```python
from build123d import *

# Parameters (mm, degrees)
SKETCH1_R               = 16
BOSS_EXTRUDE1_DEPTH     = 25
CUT_EXTRUDE1_DEPTH      = 34.7194306
CUT_EXTRUDE1_DEPTH_BACK = 34.7194306
SKETCH2_R               = 6
CUT_EXTRUDE2_START      = -4
CUT_EXTRUDE2_DEPTH      = 12


with BuildPart() as part:
    # Sketch1 → Boss-Extrude1 (new body)
    with BuildSketch(Plane.XY):
        Circle(SKETCH1_R)
    extrude(amount=-BOSS_EXTRUDE1_DEPTH)

    # Sketch2 → Cut-Extrude1 (cut, two sides: drawn at the far end of the back side and taken through both)
    with BuildSketch(Plane(origin=(0, 0, 0), x_dir=(1, 0, 0), z_dir=(0, 1, 0)).offset(-CUT_EXTRUDE1_DEPTH_BACK)):
        with Locations(Location((0, 10, 0), (0, 0, 270))):
            Circle(SKETCH2_R)
    extrude(amount=CUT_EXTRUDE1_DEPTH + CUT_EXTRUDE1_DEPTH_BACK, mode=Mode.SUBTRACT)

    # Sketch3 → Cut-Extrude2 (cut)
    with BuildSketch(Plane.XY.offset(CUT_EXTRUDE2_START)):
        with BuildLine():
            Line((-7.81200483, 11.010112649), (-9.258672391, 13.049022398))
            ThreePointArc((-9.258672391, 13.049022398), (0.598342854, 15.988808143), (10.208066995, 12.320526296))
            Line((10.208066995, 12.320526296), (8.613056527, 10.395444063))
            ThreePointArc((8.613056527, 10.395444063), (0.504851783, 13.490556871), (-7.81200483, 11.010112649))
        make_face()
    extrude(amount=-CUT_EXTRUDE2_DEPTH, mode=Mode.SUBTRACT)


solid = part.part
```
Source: CAD feature listing. Evaluate the final solid. Frame: model axes, mm. A direction names the side the tool comes from. Give positions to 0.01 mm unless a question says otherwise; leave off trailing zeros. Loops run counter-clockwise (first coordinate to the right, second up) from the corner with the lowest first, then second, coordinate; pieces in that order, holes last. Notation, with made-up numbers: (1, 69) - (50, 69) arc R23 ccw to (50, 84) - close; hole circle Ø10 at (-15, 59.5). An arc over 180 degrees is marked (long way). Use CSV: the item, a comma, the result in double quotes. Start each with the question number.
1. Draft query along X for faces 1 (the cylindrical face through (-3.47, -15.62, -15.1)), 2 (the flat face through (0, 0, 0)), 3 (the flat face through (9.42, 11.37, -9.92)). Return one class per face: +X half, -X half, draft (parallel to the pull), parting line (faces both ways), or undercut.
2. Section A-A (x = -2). Output: boundary loops of the cut face in (y, z).
3. Section D-D (x = 7). Output: boundary loops of the cut face in (y, z), then the cut area to 3 significant figures.
4. Section C-C (y = 0). Output: boundary loops of the cut face in (x, z), then the cut area to 3 significant figures.
5. Ray query, L1, parallel to Z at x = 0, y = -2.75; L2, parallel to X at y = -5.5, z = -5.5; L3, parallel to X at y = 5.5, z = -15. Return the intervals inside material, ascending.
6. Section B-B (z = -12). Output: boundary loops of the cut face in (x, y).
7. Pin query (flat end, axial travel): pin 1 (5 mm diameter, centred on y = 7, z = -7.5, fed in from +X); pin 2 (2 mm diameter, centred on y = -6.5, z = -17.5, fed in from +X) (3 decimals); pin 3 (4.5 mm diameter, centred on x = -1.5, y = 13, fed in from +Z); pin 4 (10 mm diameter, centred on y = -5.5, z = -9.5, fed in from +X). Return the tip coordinate at first contact, or that it passes through.
8. Reachability of faces 4 (the cylindrical face through (1.802, -1.462, -4.277)), 5 (the flat face through (1, 14, -4)) from +Z, -Z, +X, -X, +Y, -Y: full face, straight path, thin tool, end or side. Return the list, or none.
Response:
1,face 1,"parting line"
1,face 2,"draft"
1,face 3,"undercut"
2,outline,"(-15.87, -25) - (15.87, -25) - (15.87, -16) - (13.35, -16) - (13.35, -15.66) - (-15.87, -15.66) - close; (-15.87, -4.34) - (13.35, -4.34) - (13.35, -4) - (15.87, -4) - (15.87, 0) - (-15.87, 0) - close"
3,outline,"(-14.39, -25) - (14.39, -25) - (14.39, -16) - (11.54, -16) - (11.54, -4) - (14.39, -4) - (14.39, 0) - (-14.39, 0) - close"
3,area,"685 mm²"
4,outline,"(-16, -25) - (16, -25) - (16, 0) - (-16, 0) - close; hole circle Ø12 at (0, -10)"
4,area,"687 mm²"
5,L1,"-25 to -16, -4 to 0"
5,L2,"-15.02 to -3.97, 3.97 to 15.02"
5,L3,"-15.02 to -3.32, 3.32 to 15.02"
6,outline,"(-9.26, 13.05) arc R16 ccw to (-5.66, -14.97) - (-5.66, 12.26) arc R13.5 ccw to (-7.81, 11.01) - close; (5.66, -14.97) arc R16 ccw to (10.21, 12.32) - (8.61, 10.4) arc R13.5 ccw to (5.66, 12.26) - close"
7,pin 1,"x = 15.35"
7,pin 2,"x = 15.025"
7,pin 3,"z = 0"
7,pin 4,"x = 15.99"
8,face 4,"+Y, -Y"
8,face 5,"+Y"
